Model file for the job. Use its own axes, mm. Face numbers are marked on the shaded views. A direction names the side the tool comes from. Coordinates: 2 decimals unless noted, no trailing zeros. Write each loop counter-clockwise with the first axis right and the second up, starting at its lowest first coordinate (ties: lowest second). Pieces come first, ordered by that corner, then holes.
Q1. Drill centre lines: probe 1 along Z at (x, y) = (14.75, 12.1); probe 2 along X at (y, z) = (11, -24.5); probe 3 along Y at (x, z) = (3.5, -15.5). Where is each one in solid material? Low to high.
Q2. Band-saw the part on C-C, the plane z = -5. Write the cut outline in (x, y).
Q3. Which spindle directions (+Z, -Z, +X, -X, +Y, -Y) get a long thin tool onto all of the face, cutting with end or side? Do the marked faces 1, 2 and 3. Say none if no direction does.
Q4. Band-saw the part on D-D, the plane y = 1. Write the cut outline in (x, z), plus the area to 3 significant figures.
Q5. Band-saw the part on B-B, the plane y = 7.1. Write the cut outline in (x, z).
Q6. Band-saw the part on A-A, the plane y = 20.1. Write the cut outline in (x, z), plus the area to 3 significant figures.
Q7. Pin check, flat tips, straight feed: P1, Ø6, axis at x = 3, z = -8, coming from the +Y side; P2, Ø4.5, axis at x = 8, z = -21, coming from the -Y side; P3, Ø6, axis at y = 34, z = -18.5, coming from the -X side. Stop position of each tip, or through.
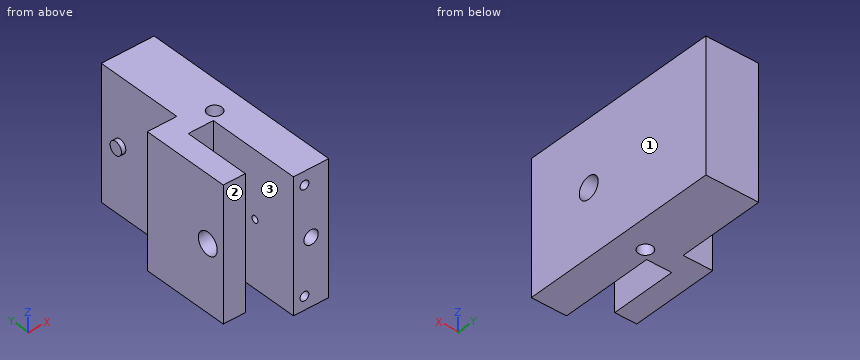
Autodesk Inventor part; units mm, degrees
ref_plane "YZ Plane" through (0, 0, 0) normal (1, 0, 0) x (0, 1, 0)
ref_plane "XZ Plane" through (0, 0, 0) normal (0, 1, 0) x (-1, 0, 0)
ref_plane "XY Plane" through (0, 0, 0) normal (0, 0, 1) x (1, 0, 0)
ref_plane "Arbeitsebene1" through (0, 0, 0) normal (0, 0, -1) x (-1, 0, 0)
sketch "Skizze1" plane through (0, 0, 0) normal (0, 0, -1) x (-1, 0, 0)
  line L0 (-9, -16) -> (-9, 16) construction
  line L1 (-9, 16) -> (-7.5, 16) construction
  line L2 (-7.5, -1) -> (-7.5, -16) construction
  line L3 (-11.1, -3.1) -> (-19.1, -3.1) construction
  line L4 (-19.1, -3.1) -> (-19.1, 43.1)
  line L5 (-19.1, 43.1) -> (-7.1, 43.1)
  line L6 (-7.1, 23.1) -> (-0.4, 23.1)
  line L7 (-0.4, 23.1) -> (-0.4, 3)
  line L8 (-0.4, 3) -> (-5.4, 3)
  line L9 (-5.4, 3) -> (-5.4, 18.1)
  line L10 (-5.4, 18.1) -> (-11.1, 18.1)
  line L11 (-11.1, 18.1) -> (-11.1, -3.1)
  line L12 (-19.1, -3.1) -> (-11.1, -3.1)
  line L13 (-11.1, -3.1) -> (-9, -3.1) construction
  line L14 (-9, 18.1) -> (-9, 16) construction
  line L15 (-7.5, 16) -> (-5.4, 16) construction
  line L16 (-7.1, 23.1) -> (-7.1, 43.1)
  point P0 (0, 0)
  dimension "d0" = 20
  dimension "d1" = 5
  dimension "d2" = 5
  dimension "d3" = 13
  dimension "d18" = 12
extrude "Extrusion1" add sketch "Skizze1" along normal blind 30
sketch "Skizze2" plane through (7.1, 23.1, 0) normal (-1, 0, 0) x (0, 0, 1)
  line L0 (0, 20) -> (-30, 20)
  line L1 (-15, 15) -> (-15, 20) construction
  circle A0 centre (-15, 15) radius 1.5
  point P0 (0, -23.1)
  point P1 (-15, 20)
  point P2 (-15, 20)
  dimension "d6" = 5
  dimension "d94" = 3
sketch "Skizze3" plane through (11.1, -3.1, 0) normal (0, -1, 0) x (1, 0, 0)
  circle A0 centre (4, -15) radius 2 construction
  point P0 (-11.1, 0)
hole "Katzeverbindung" at (15.1, -3.1, -15) direction (0, 1, 0) diameter 3.242 depth 11.8 tip angle 118
sketch "Skizze4" plane through (11.1, -3.1, 0) normal (0, -1, 0) x (1, 0, 0)
  circle A0 centre (2.5, -27) radius 1
  circle A1 centre (2.5, -3) radius 1
  point P0 (-11.1, 0)
hole "Zentrierbolzen" at (13.6, -3.1, -3) at (13.6, -3.1, -27) direction (0, 1, 0) diameter 2 depth 6 tip angle 118
sketch "Skizze5" plane through (0, 0, 0) normal (0, 0, 1) x (1, 0, 0)
  line L0 (19.1, 43.1) -> (19.1, -3.1)
  line L1 (7.1, 43.1) -> (19.1, 43.1)
  point P0 (0, 0)
  point P1 (13.1, 20.1)
  dimension "d92" = 6
  dimension "d93" = 23
hole "seilV" at (13.1, 20.1, 0) direction (0, 0, -1) diameter 3.242 end through all
sketch "Skizze6" plane through (5.4, 18.1, 0) normal (0, -1, 0) x (1, 0, 0)
  line L0 (5.7, 0) -> (0, 0) construction
  line L1 (0, 0) -> (0, -30) construction
  line L2 (5.7, -30) -> (0, -30) construction
  line L3 (5.7, 0) -> (5.7, -30) construction
  line L4 (5.7, -15) -> (2.85, -15) construction
  line L5 (2.85, -15) -> (2.85, -30) construction
  line L6 (2.85, -15) -> (2.85, 0) construction
  line L7 (2.85, -15) -> (0, -15) construction
  line L8 (5.7, 0) -> (5.7, -30) construction
  point P0 (-5.4, 0)
hole "GLVV" at (8.25, 18.1, -15) direction (0, 1, 0) diameter 1.567 depth 4 tip angle 118
sketch "Skizze7" plane through (11.1, -3.1, 0) normal (-1, 0, 0) x (0, 0, 1)
  line L0 (-30, 19.2) -> (0, 19.2) construction
  line L1 (0, 0) -> (0, 21.2) construction
  line L2 (0, 21.2) -> (-30, 21.2) construction
  line L3 (-30, 0) -> (-30, 21.2) construction
  line L4 (0, 0) -> (-30, 0) construction
  line L5 (-30, 10.2) -> (-15, 10.2) construction
  line L6 (-15, 10.2) -> (0, 10.2) construction
  line L7 (-15, 10.2) -> (-15, 19.2) construction
  point P0 (0, 3.1)
  dimension "d62" = 9
hole "GLVO" at (11.1, 7.1, -15) direction (1, 0, 0) diameter 1.567 depth 4 tip angle 118
sketch "Skizze8" plane through (5.4, 3, 0) normal (1, 0, 0) x (0, 0, -1)
  line L0 (0, 15.1) -> (0, 0) construction
  line L1 (0, 0) -> (30, 0) construction
  line L2 (30, 15.1) -> (30, 0) construction
  line L3 (0, 15.1) -> (30, 15.1) construction
  line L4 (0, 13.1) -> (30, 13.1) construction
  line L5 (15, 9.1) -> (15, 13.1) construction
  line L6 (15, 9.1) -> (0, 9.1) construction
  line L7 (15, 9.1) -> (30, 9.1) construction
  line L8 (30, 15.1) -> (30, 0) construction
  point P0 (0, -3)
  dimension "d70" = 4
hole "GLVU" at (5.4, 12.1, -15) direction (-1, 0, 0) diameter 1.567 depth 4 tip angle 118
sketch "Skizze9" plane through (0.4, 3, 0) normal (-1, 0, 0) x (0, 0, 1)
  circle A0 centre (-15, 4.1) radius 1
  point P0 (0, -3)
hole "DLVU" at (0.4, 7.1, -15) direction (1, 0, 0) diameter 5 depth 5
sketch "Skizze10" plane through (11.1, -3.1, 0) normal (-1, 0, 0) x (0, 0, 1)
  circle A0 centre (-15, 15.2) radius 0.7835
  point P0 (0, 3.1)
hole "DLVO" at (11.1, 12.1, -15) direction (1, 0, 0) diameter 5 end through all
extrude "Extrusion2" add sketch "Skizze2" along normal blind 1
properties part number "Katze_Lagerhalter_vorne" material "Aluminium 6061, Katze"
Answer sheet:
1. probe 1: z = -30 to -17.5, -12.5 to 0
1. probe 2: x = 0.4 to 5.4, 11.1 to 19.1
1. probe 3: y = 3 to 4.65, 9.55 to 11.5, 12.7 to 23.1
2. outline: (0.4, 3) - (5.4, 3) - (5.4, 18.1) - (11.1, 18.1) - (11.1, -3.1) - (19.1, -3.1) - (19.1, 43.1) - (7.1, 43.1) - (7.1, 23.1) - (0.4, 23.1) - close; hole circle Ø3.24 at (13.1, 20.1)
3. face 1: +Z, -Z, +X, +Y, -Y
3. face 2: +Z, -Z, -X, -Y
3. face 3: +Z, -Z, -Y
4. outline: (11.1, -30) - (19.1, -30) - (19.1, 0) - (11.1, 0) - close; hole circle Ø2 at (13.6, -27); hole circle Ø2 at (13.6, -3); hole circle Ø3.24 at (15.1, -15)
4. area: 225 mm2
5. outline: (0.4, -30) - (5.4, -30) - (5.4, -17.5) - (0.4, -17.5) - close; (0.4, -12.5) - (5.4, -12.5) - (5.4, 0) - (0.4, 0) - close; (11.1, -30) - (19.1, -30) - (19.1, 0) - (11.1, 0) - (11.1, -14.22) - (13.68, -14.22) arc R1.62 cw (long way) to (13.68, -15.78) - (11.1, -15.78) - close
6. outline: (0.4, -30) - (11.48, -30) - (11.48, 0) - (0.4, 0) - close; (14.72, -30) - (19.1, -30) - (19.1, 0) - (14.72, 0) - close; hole circle Ø1.57 at (8.25, -15)
6. area: 462 mm2
7. P1: stops at y = 23.1
7. P2: stops at y = 18.1
7. P3: stops at x = 7.1
